Source: CAD feature listing. Evaluate the final solid. Frame: model axes, mm. A direction names the side the tool comes from. Coordinates: 2 decimals unless noted, no trailing zeros. Write each loop counter-clockwise with the first axis right and the second up, starting at its lowest first coordinate (ties: lowest second). Pieces come first, ordered by that corner, then holes. Notation, with made-up numbers: M 43.5,44 L 90.5,44 A22 cw 90.5,54 Z; hole C 26,9 d8. An arc over 180 degrees is marked long. One line per item, written item: value. Start each with the question number.
Item 1: Cut plane D-D, the plane z = 11.25. Output: boundary loops of the cut face in (x, y).
Item 2: Pin query (flat end, axial travel): P1, Ø1.5, axis at x = 1, y = 1.5, coming from the -Z side; P2, Ø2, axis at x = 1.5, z = 6, coming from the -Y side. Return the tip coordinate at first contact, or that it passes through.
Item 3: Cut plane B-B, the plane y = 0. Output: boundary loops of the cut face in (x, z).
Item 4: Set-up query: faces 4 (the flat face through (-0.2, -4.3, 12)), 5 (the flat face through (4, 0, 6)), 6 (the flat face through (1.4, -7, 4.6)). Return all of +Z, -Z, +X, -X, +Y, -Y with unobstructed straight access to the full face (end or side cutting, diameter ignored); none if empty.
Item 5: Cut plane A-A, the plane x = 0. Output: boundary loops of the cut face in (y, z), then the cut area to 3 significant figures.
Item 6: Mould query, pull axis Z, two halves, no side actions, for faces 1 (the flat face through (-0.2, -4.3, 0)), 2 (the cylindrical face through (5.631, -9.725, 6.084)), 3 (the cylindrical face through (1.75, -8.52, 8.74)). Classes: released by +Z, released by -Z, zero draft, split by the parting line, or undercut.
Item 7: Cut plane C-C, the plane z = 6. Output: boundary loops of the cut face in (x, y).
Item 8: Ray query, L1, parallel to Y at x = -2.75, z = 11; L2, parallel to Z at x = 0, y = -8.1; L3, parallel to Z at x = 0, y = -4.95. Return the intervals inside material, ascending. Write a range as from..to.
```python
from build123d import *

# Parameters (mm, degrees)
F0_W           = 8
F0_H           = 8
F1_DEPTH       = 12
F3_D           = 3.3
F3_DEPTH       = 12
F3_CBORE_D     = 6.5
F3_CBORE_DEPTH = 3
F3_TIP         = 0.9914200214
F4_R           = 2


with BuildPart() as f1:
    # F0 (on Top) → F1 (new body)
    with BuildSketch(Plane.XY):
        Polygon((5.7735026919, -10), (11.5470053838, 0), (5.7735026919, 10), (-5.7735026919, 10), (-11.5470053838, 0), (-5.7735026919, -10), align=None)
        Rectangle(F0_W, F0_H, mode=Mode.SUBTRACT)
    extrude(amount=F1_DEPTH)

    # F3
    with Locations(Plane.XZ.offset(10)):
        with Locations((0, 6)):
            CounterBoreHole(F3_D / 2, F3_CBORE_D / 2, F3_CBORE_DEPTH, depth=F3_DEPTH)
            with Locations((0, 0, -(F3_DEPTH + F3_TIP / 2))):  # 118° drill point
                Cone(0, F3_D / 2, F3_TIP, mode=Mode.SUBTRACT)

    # F4
    f4_edges = [f1.edges().sort_by_distance(p)[0] for p in [
        (-11.547005, 0, 6),
        (-5.773503, -10, 6),
        (5.773503, -10, 6),
        (11.547005, 0, 6),
        (5.773503, 10, 6),
        (-5.773503, 10, 6),
    ]]
    fillet(f4_edges, radius=F4_R)


solid = f1.part
```
From the geometry:
1. outline: M -10.97,-1 L -6.35,-9 A2 ccw -4.62,-10 L 4.62,-10 A2 ccw 6.35,-9 L 10.97,-1 A2 ccw 10.97,1 L 6.35,9 A2 ccw 4.62,10 L -4.62,10 A2 ccw -6.35,9 L -10.97,1 A2 ccw Z; hole M -4,-4 L 4,-4 L 4,4 L -4,4 Z
2. P1: passes through
2. P2: stops at y = -7
3. outline: M -11.24,0 L -4,0 L -4,12 L -11.24,12 Z; M 4,0 L 11.24,0 L 11.24,12 L 4,12 Z
4. face 4: +Z, +X, -X, +Y, -Y
4. face 5: +Z, -Z
4. face 6: -Y
5. outline: M -10,0 L -4,0 L -4,4.35 L -7,4.35 L -7,2.75 L -10,2.75 Z; M -10,9.25 L -7,9.25 L -7,7.65 L -4,7.65 L -4,12 L -10,12 Z; M 4,0 L 10,0 L 10,12 L 4,12 Z
5. area: 115 mm²
6. face 1: released by -Z
6. face 2: zero draft
6. face 3: undercut
7. outline: M -10.97,-1 L -6.35,-9 A2 ccw -4.62,-10 L -3.25,-10 L -3.25,-7 L -1.65,-7 L -1.65,-4 L -4,-4 L -4,4 L 4,4 L 4,-4 L 1.65,-4 L 1.65,-7 L 3.25,-7 L 3.25,-10 L 4.62,-10 A2 ccw 6.35,-9 L 10.97,-1 A2 ccw 10.97,1 L 6.35,9 A2 ccw 4.62,10 L -4.62,10 A2 ccw -6.35,9 L -10.97,1 A2 ccw Z
8. L1: y = -10..-4, 4..10
8. L2: z = 0..2.75, 9.25..12
8. L3: z = 0..4.35, 7.65..12
